from build123d import *

# Parameters (mm, degrees)
CUT_EXTRUDE1_DEPTH = 1.4


with BuildPart() as part:
    # Sketch2 → Revolve1 (revolve)
    with BuildSketch(Plane(origin=(0, 0, 0), x_dir=(0, 0, -1), z_dir=(1, 0, 0)), mode=Mode.PRIVATE) as revolve1_sk:
        with BuildLine():
            Line((-7.825, 0), (7.825, 0))
            Line((7.825, 0), (7.825, 1.1))
            Line((7.825, 1.1), (7.425, 1.5))
            Line((7.425, 1.5), (-6.175, 1.5))
            Line((-6.175, 1.5), (-6.175, 2.85))
            Line((-6.175, 2.85), (-6.4225, 2.85))
            ThreePointArc((-6.4225, 2.85), (-7.22987489, 2.285251969), (-7.825, 1.5))
            Line((-7.825, 1.5), (-7.825, 0))
        make_face()
    revolve(revolve1_sk.sketch.rotate(Axis((0, 0, 7.825), (0, 0, -1)), 90), axis=Axis((0, 0, 7.825), (0, 0, -1)))

    # Sketch3 → Cut-Extrude1 (cut)
    with BuildSketch(Plane.XY.offset(7.825)):
        Polygon((0, 1.154700538), (-1, 0.577350269), (-1, -0.577350269), (0, -1.154700538), (1, -0.577350269), (1, 0.577350269), align=None)
    extrude(amount=-CUT_EXTRUDE1_DEPTH, mode=Mode.SUBTRACT)

    # Cut-Extrude2 cone 1 section (through the dimple's axis) → Cut-Extrude2 (revolve, cut)
    with BuildSketch(Plane(origin=(0, 0, 7.825), x_dir=(0, -1, 0), z_dir=(1, 0, 0))):
        Polygon((0, 0), (1.154700538, 0), (0, 1.154700538), align=None)
    revolve(axis=Axis((0, 0, 7.825), (0, 0, -1)), mode=Mode.SUBTRACT)


solid = part.part
Source: CAD feature listing. Evaluate the final solid. Frame: model axes, mm. A direction names the side the tool comes from. Coordinates: 2 decimals unless noted, no trailing zeros. Loops run counter-clockwise (first coordinate to the right, second up) from the corner with the lowest first, then second, coordinate; pieces in that order, holes last. Notation, with made-up numbers: (63, 10.5) - (78, 10.5) arc R22 ccw to (78, 24.5) - close; hole circle Ø4 at (83.25, -40). An arc over 180 degrees is marked (long way). One line per item, written item: value. Start each with the question number.
1. Mould query, pull axis X, two halves, no side actions, for faces 1 (the cylindrical face through (1.43, -0.45, -0.53)), 2 (the flat face through (-1, 0, 7)), 3 (the flat face through (0, 0, -7.825)), 4 (the flat face through (-0.49, 0.87, 7.13)). Classes: pulls with the +X half, pulls with the -X half, needs draft (parallel to the pull), parting line crosses it, or undercut.
2. Ray query, L1, parallel to Z at x = 0, y = 0.5 (3 decimals); L2, parallel to X at y = 0.8, z = -3; L3, parallel to Y at x = 0.05, z = 0. Return the intervals inside material, ascending.
3. Set-up query: faces 5 (the flat face through (-0.51, -0.86, 7.13)), 6 (the flat face through (-1.2, 1.2, 6.175)). Return all of +Z, -Z, +X, -X, +Y, -Y with unobstructed straight access to the full face (end or side cutting, diameter ignored); none if empty.
4. Contact query for flat-ended pins moving along their axis: P1, Ø1, axis at x = 0, y = -0.5, coming from the +Z side (3 decimals); P2, Ø3, axis at x = -1, z = 1.5, coming from the +Y side; P3, Ø1, axis at y = 1.5, z = 3.5, coming from the -X side. Output: stop coordinate, or through.
5. Section B-B (z = -1.75). Return the cut outline in (x, y).
Verdict:
1. face 1: parting line crosses it
1. face 2: undercut
1. face 3: needs draft
1. face 4: undercut
2. L1: z = -7.825 to 6.425
2. L2: x = -1.27 to 1.27
2. L3: y = -1.5 to 1.5
3. face 5: +Z
3. face 6: -Z
4. P1: stops at z = 6.425
4. P2: stops at y = 1.5
4. P3: stops at x = -1.12
5. outline: circle Ø3 at (0, 0)
